```python
from build123d import *

# Parameters (mm, degrees)
SKETCH1_W                  = 54.5
SKETCH1_H                  = 111
BOSS_EXTRUDE1_DEPTH        = 4.5
SKETCH2_W                  = 13.5
SKETCH2_H                  = 111
BOSS_EXTRUDE2_DEPTH        = 12.5
M4X0_7_TAPPED_HOLE1_D      = 3.3
SKETCH6_W                  = 4
SKETCH6_H                  = 12.5
BOSS_EXTRUDE3_DEPTH        = 37
SKETCH7_W                  = 54.5
SKETCH7_H                  = 3
BOSS_EXTRUDE5_DEPTH        = 39
SKETCH8_R                  = 7
CUT_EXTRUDE1_DEPTH         = 3
M2_CLEARANCE_HOLE1_D       = 2.4
F_8_0_199_DIAMETER_HOLE1_D = 5.0546
SKETCH12_R                 = 5.5
CUT_EXTRUDE3_DEPTH         = 3


with BuildPart() as part:
    # Sketch1 → Boss-Extrude1 (new body)
    with BuildSketch(Plane(origin=(0, 0, 0), x_dir=(1, 0, 0), z_dir=(0, 1, 0))):
        with Locations((-13.399543841, 44.129312584)):
            Rectangle(SKETCH1_W, SKETCH1_H)
    extrude(amount=BOSS_EXTRUDE1_DEPTH)

    # Sketch2 → Boss-Extrude2 (add)
    with BuildSketch(Plane(origin=(0, 4.5, 0), x_dir=(1, 0, 0), z_dir=(0, 1, 0))):
        with Locations((7.100456159, 44.129312584)):
            Rectangle(SKETCH2_W, SKETCH2_H)
        with Locations((-33.899543841, 44.129312584)):
            Rectangle(SKETCH2_W, SKETCH2_H)
    extrude(amount=BOSS_EXTRUDE2_DEPTH)

    # M4x0.7 Tapped Hole1 (through all)
    with Locations(Plane(origin=(-31.949543841, 17, -9.129312584), x_dir=(0, 0, 1), z_dir=(0, 1, 0))):
        with Locations((0, 0), (-25, 0), (-50, 0), (-75, 0), (0, 37.1), (-25, 37.1), (-50, 37.1), (-75, 37.1)):
            Hole(M4X0_7_TAPPED_HOLE1_D / 2)

    # Sketch6 → Boss-Extrude3 (add)
    with BuildSketch(Plane(origin=(-27.149543841, 0, 0), x_dir=(0, 0, -1), z_dir=(1, 0, 0))):
        with Locations((-9.370687416, 10.75)):
            Rectangle(SKETCH6_W, SKETCH6_H)
    extrude(amount=BOSS_EXTRUDE3_DEPTH)

    # Sketch7 → Boss-Extrude5 (add)
    with BuildSketch(Plane.XY.offset(11.370687416)):
        with Locations((-13.399543841, 15.5)):
            Rectangle(SKETCH7_W, SKETCH7_H)
    extrude(amount=BOSS_EXTRUDE5_DEPTH)

    # Sketch8 → Cut-Extrude1 (cut)
    with BuildSketch(Plane(origin=(0, 17, 0), x_dir=(1, 0, 0), z_dir=(0, 1, 0))):
        with Locations((-13.399543841, -30.870687416)):
            Circle(SKETCH8_R)
    extrude(amount=-CUT_EXTRUDE1_DEPTH, mode=Mode.SUBTRACT)

    # M2 Clearance Hole1 (through all)
    with Locations(Plane(origin=(-21.371437118, 17, 30.847906254), x_dir=(0, 0, 1), z_dir=(0, 1, 0))):
        with Locations((0, 0), (-7.977218838, 7.971893277), (8.022781162, 7.971893277), (-0.002806072, 15.940961576)):
            Hole(M2_CLEARANCE_HOLE1_D / 2)

    # #8 (0.199) Diameter Hole1 (through all)
    with Locations(Plane(origin=(-13.399543841, 4.5, 2.370687416), x_dir=(0, 0, 1), z_dir=(0, 1, 0))):
        with Locations((0, 0), (-10, 0), (-35, 0), (-85, 0), (-95, 0)):
            Hole(F_8_0_199_DIAMETER_HOLE1_D / 2)

    # Sketch12 → Cut-Extrude3 (cut)
    with BuildSketch(Plane(origin=(0, 0, 0), x_dir=(-1, 0, 0), z_dir=(0, -1, 0))):
        with Locations((13.399543841, 92.629312584)):
            Circle(SKETCH12_R)
    extrude(amount=-CUT_EXTRUDE3_DEPTH, mode=Mode.SUBTRACT)


solid = part.part
```
The model under review builds one solid part; all positions refer to its coordinate system, in mm. A direction names the side the tool comes from. Round coordinates to 2 decimals unless told otherwise and drop trailing zeros. Loops run counter-clockwise (first coordinate to the right, second up) from the corner with the lowest first, then second, coordinate; pieces in that order, holes last.
1) Consider section A-A on y = 7.75. Give the number of separate pieces and of enclosed holes in the cut face, then the cut area to 3 significant figures.
Values follow:
separate pieces: 1
enclosed holes: 8
area: 3,040 mm2
2) Consider section B-B on x = -35.5. State the section outline as (y, z) points.
Values follow:
outline: (0, -99.63) - (17, -99.63) - (17, 50.37) - (14, 50.37) - (14, 11.37) - (0, 11.37) - close
3) Consider section D-D on z = 15. State the section outline as (x, y) points, then the cut area to 4 significant figures.
Values follow:
outline: (-40.65, 14) - (13.85, 14) - (13.85, 17) - (-40.65, 17) - close
area: 163.5 mm2
4) Consider section C-C on z = -59. State the section outline as (x, y) points.
Values follow:
outline: (-40.65, 0) - (-33.59, 0) - (-33.59, 17) - (-40.65, 17) - close; (-30.3, 0) - (3.51, 0) - (3.51, 17) - (0.35, 17) - (0.35, 4.5) - (-27.15, 4.5) - (-27.15, 17) - (-30.3, 17) - close; (6.8, 0) - (13.85, 0) - (13.85, 17) - (6.8, 17) - close
5) The part is to be moulded in two halves that separate along X. For faces 1 (the face through (6.266, 8.381, -7.913)), 2 (the face through (-40.65, 8, -42)), 3 (the face through (-14, 3, -99.629)), 4 (the face through (13.85, 8, -42)), say which applies: pulls with the +X half, pulls with the -X half, needs draft (parallel to the pull), parting line crosses it, or undercut.
Values follow:
face 1: undercut
face 2: pulls with the -X half
face 3: needs draft
face 4: pulls with the +X half
6) Wall thickness on line 1 along X through (y, z) = (13.75, -12); line 2 along Z through (x, y) = (4, 1); line 3 along Y through (x, z) = (-15.5, -26): over which ranges is each line inside the solid? List them lowest first.
Values follow:
line 1: x = -40.65 to -27.15, 0.35 to 13.85
line 2: z = -99.63 to -85.31, -82.95 to -60.31, -57.95 to -35.31, -32.95 to -10.31, -7.95 to 11.37
line 3: y = 0 to 4.5
7) Tool access review of faces 5 (the face through (-18.28, 15.52, 25.85)), 6 (the face through (-14, 7, 11.371)), 7 (the face through (-16, 3, -91)), 8 (the face through (0.35, 11, -45)): name each direction out of +Z, -Z, +X, -X, +Y, -Y from which nothing blocks a thin tool from reaching the whole face with its end or side.
Values follow:
face 5: +Y, -Y
face 6: +Z, +X, -X, -Y
face 7: -Y
face 8: -Z, +Y
8) Clearance check with flat-ended pins moving along their axes: P1, Ø3, axis at x = -13.4, z = 38.87, coming from the -Y side; P2, Ø6.5, axis at x = -13.4, z = -82.63, coming from the +Y side; P3, Ø8, axis at x = -30, y = 4.5, coming from the +Z side. State where each tip first meets the part, or that it passes through.
Values follow:
P1: stops at y = 14
P2: stops at y = 4.5
P3: stops at z = 11.37
